The drawing under review shows one solid part. Ordinate dimensions are in mm from its lowest x, y, z. Give positions to 0.01 mm unless a question says otherwise; leave off trailing zeros. Loops run counter-clockwise (first coordinate to the right, second up) from the corner with the lowest first, then second, coordinate; pieces in that order, holes last. Notation, with made-up numbers: (-15.75, 79.25) -> (17.25, 79.25) arc R32 ccw to (17.25, 116.25) -> close; hole circle Ø2 at (61.25, -16.75). An arc over 180 degrees is marked (long way). Answer in a Markdown table with one row per item. Add a question column.
(1) For line 1 (Z direction, x = 10, y = 1.45); line 2 (X direction, y = 1.35, z = 7); line 3 (Z direction, x = 8, y = 0.25) (1 decimal), list the stretches that pass through material, from the lowest coordinate up.
(2) Consider section D-D on x = 5.5. Write out the cut boundary in (y, z).
(3) Draft analysis for pull direction Y (two halves, no side actions). For the marked faces 1 and 2, state which applies: +Y half, -Y half, draft (parallel to the pull), parting line (faces both ways), or undercut.
(4) Consider section A-A on y = 0.75. Write out the cut boundary in (x, z), then the cut area to 3 significant figures.
(5) Consider section C-C on z = 3. Write out the cut boundary in (x, y).
(6) Consider section B-B on x = 10. Write out the cut boundary in (y, z), then the cut area to 3 significant figures.
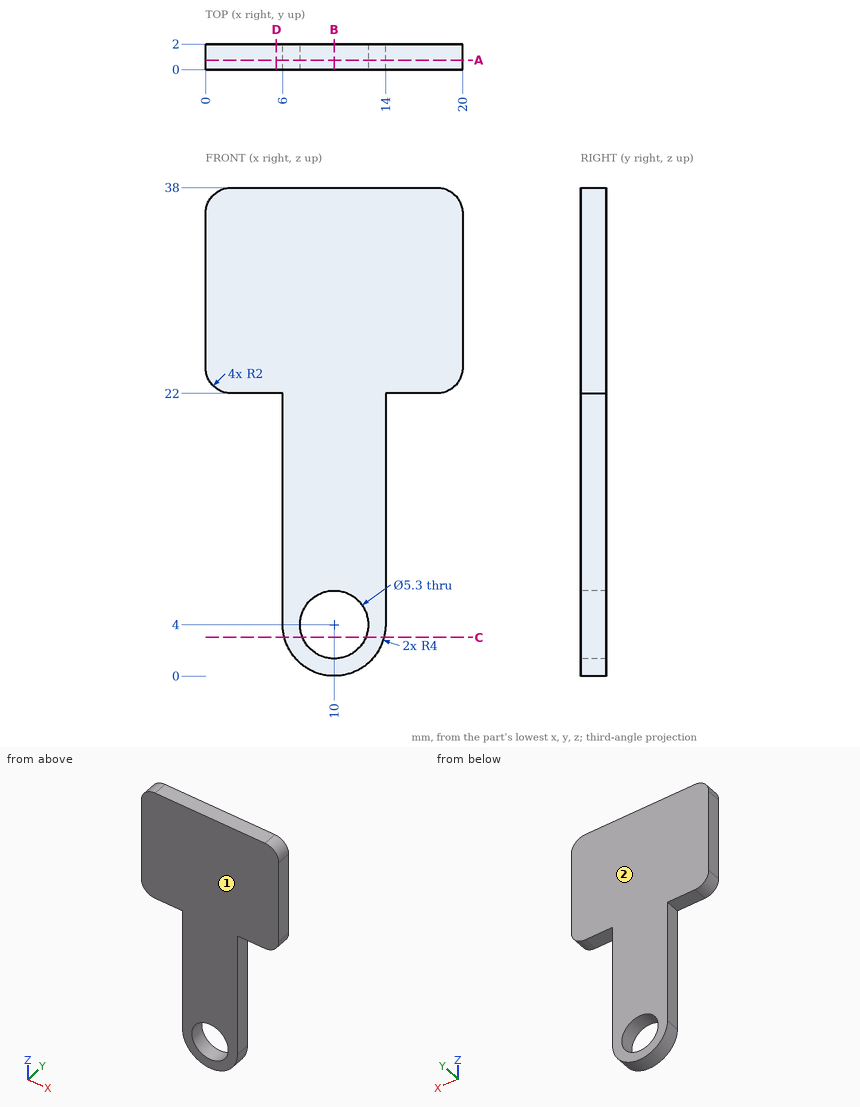
Values follow:
| question | item | result |
|---|---|---|
| 1 | line 1 | 0 to 1.35, 6.65 to 38 |
| 1 | line 2 | 6 to 14 |
| 1 | line 3 | 0.5 to 2.3, 5.7 to 38 |
| 2 | outline | (0, 22) -> (2, 22) -> (2, 38) -> (0, 38) -> close |
| 3 | face 1 | -Y half |
| 3 | face 2 | +Y half |
| 4 | outline | (0, 24) arc R2 ccw to (2, 22) -> (6, 22) -> (6, 4) arc R4 ccw to (13.27, 1.69) arc R4 ccw to (14, 4) -> (14, 22) -> (18, 22) arc R2 ccw to (20, 24) -> (20, 36) arc R2 ccw to (18, 38) -> (2, 38) arc R2 ccw to (0, 36) -> close; hole circle Ø5.3 at (10, 4) |
| 4 | area | 464 mm2 |
| 5 | outline | (6.13, 0) -> (7.55, 0) -> (7.55, 2) -> (6.13, 2) -> close; (12.45, 0) -> (13.87, 0) -> (13.87, 2) -> (12.45, 2) -> close |
| 6 | outline | (0, 0) -> (2, 0) -> (2, 1.35) -> (0, 1.35) -> close; (0, 6.65) -> (2, 6.65) -> (2, 38) -> (0, 38) -> close |
| 6 | area | 65.4 mm2 |
